Autodesk Inventor part; units mm, degrees
ref_plane "YZ Plane" through (0, 0, 0) normal (1, 0, 0) x (0, 1, 0)
ref_plane "XZ Plane" through (0, 0, 0) normal (0, 1, 0) x (-1, 0, 0)
ref_plane "XY Plane" through (0, 0, 0) normal (0, 0, 1) x (1, 0, 0)
sketch "Skizze1" plane through (0, 0, 0) normal (0, 0, 1) x (1, 0, 0)
  line L0 (-36.5, 103.5) -> (36.5, 103.5)
  line L1 (36.5, 103.5) -> (36.5, -103.5)
  line L2 (36.5, -103.5) -> (-36.5, -103.5)
  line L3 (-36.5, -103.5) -> (-36.5, 103.5)
  point P0 (0, 0)
  point P1 (0, 103.5)
  point P2 (-36.5, 0)
  dimension "d0" = 73
  dimension "d1" = 207
extrude "Extrusion1" add sketch "Skizze1" along normal mid plane 71
sketch "Skizze2" plane through (0, 0, 35.5) normal (0, 0, 1) x (1, 0, 0)
  line L0 (-31.9691, 54.6598) -> (-31.9691, 32.0411)
  line L1 (-31.9691, 32.0411) -> (-18.3639, 32.0411)
  line L2 (-18.3639, 32.0411) -> (-18.3639, 54.6598)
  line L3 (-18.3639, 54.6598) -> (-22.1053, 54.6598)
  line L4 (-22.1053, 54.6598) -> (-22.1053, 35.4424)
  line L5 (-22.1053, 35.4424) -> (-28.2277, 35.4424)
  line L6 (-28.2277, 35.4424) -> (-28.2277, 54.6598)
  line L7 (-28.2277, 54.6598) -> (-31.9691, 54.6598)
  line L8 (-12.2415, 54.6598) -> (-12.2415, 32.0411)
  line L9 (-12.2415, 32.0411) -> (-8.8402, 32.0411)
  line L10 (-8.8402, 32.0411) -> (-8.8402, 40.7145)
  line L11 (-8.8402, 40.7145) -> (-1.8675, 40.7145)
  line L12 (-1.8675, 40.7145) -> (-1.8675, 32.0411)
  line L13 (-1.8675, 32.0411) -> (1.7039, 32.0411)
  line L14 (1.7039, 32.0411) -> (1.7039, 54.6598)
  line L15 (1.7039, 54.6598) -> (-1.8675, 54.6598)
  line L16 (-1.8675, 45.0511) -> (-1.8675, 54.6598)
  line L17 (-1.8675, 45.0511) -> (-8.8402, 45.0511)
  line L18 (-8.8402, 45.0511) -> (-8.8402, 54.6598)
  line L19 (-12.2415, 54.6598) -> (-8.8402, 54.6598)
  line L20 (7.316, 54.6598) -> (7.316, 51.0885)
  line L21 (7.316, 51.0885) -> (12.0779, 51.0885)
  line L22 (12.0779, 51.0885) -> (12.0779, -18.2168)
  line L23 (12.0779, -18.2168) -> (19.2206, -18.2168)
  line L24 (19.2206, -18.2168) -> (19.2206, 51.0885)
  line L25 (19.2206, 51.0885) -> (23.6423, 51.0885)
  line L26 (23.6423, 51.0885) -> (23.6423, 54.6598)
  line L27 (23.6423, 54.6598) -> (7.316, 54.6598)
  line L28 (1.7039, 22.5174) -> (1.7039, 15.0346)
  line L29 (1.7039, 15.0346) -> (29.5946, 15.0346)
  line L30 (29.5946, 15.0346) -> (29.5946, 22.5174)
  line L31 (29.5946, 22.5174) -> (1.7039, 22.5174)
  line L32 (1.7039, -3.1128) -> (29.5946, -3.1128)
  line L33 (29.5946, -3.1128) -> (29.5946, -9.8501)
  line L34 (29.5946, -9.8501) -> (1.7039, -9.8501)
  line L35 (1.7039, -9.8501) -> (1.7039, -3.1128)
  point P0 (0, 0)
  point P1 (12.0779, 22.5174)
  point P2 (12.0779, 15.0346)
  point P3 (19.2206, 15.0346)
  point P4 (19.2206, 22.5174)
  point P5 (19.2206, -3.1128)
  point P6 (19.2206, -9.8501)
  point P7 (12.0779, -9.8501)
  point P8 (12.0779, -3.1128)
extrude "Extrusion2" cut sketch "Skizze2" against normal blind 0.1
chamfer "Fase1" distance 71 angle 15 1 edges at (0, 103.5, 35.5) measured on face at (12.1667, 103.5, -11.8333)
sketch "Skizze3" plane through (-36.5, 84.4756, 35.5) normal (0, 0.9659, 0.2588) x (1, 0, 0)
  circle A0 centre (36.5, 22.9067) radius 15.376
  point P0 (36.5, 12.4265)
extrude "Extrusion3" add sketch "Skizze3" along normal blind 10
properties part number "milch"
Can you work these out from the model? Positions are in its coordinate system, mm. Coordinates: 2 decimals unless noted, no trailing zeros. Loops run counter-clockwise (first coordinate to the right, second up) from the corner with the lowest first, then second, coordinate; pieces in that order, holes last. Notation, with made-up numbers: M 73,37 L 80,37 A15 ccw 80,43 Z; hole C -21,78.25 d10. An arc over 180 degrees is marked long. Return JSON: item names as keys, results as strings. Group by question number.
Item 1: I'm going to push flat-ended pins straight in: pin 1 Ø1.5 at (x, z) = (-27.5, 9.5) entering from +Y; pin 2 Ø6 at (x, z) = (6.5, 17) entering from +Y; pin 3 Ø1 at (x, z) = (-7, -27) entering from +Y. Where does each tip first touch, or does it pass through?
Item 2: Thinking about a two-plate mould opening in Z: for faces 1 (the flat face through (0.51, 95.97, -7.39)), 2 (the flat face through (-1, 1, -35.5)), 3 (the flat face through (36.5, 1, 0)), 4 (the flat face through (-30, 44, 35.4)), which applies, released by +Z, released by -Z, zero draft, split by the parting line, or undercut?
Item 3: If I drill on L1, parallel to Z at x = 15, y = -10.5; L2, parallel to Y at x = -2.5, z = 33.5; L3, parallel to Y at x = -29.5, z = 20.5, over which ranges is the centre line in solid material (lowest first)? Write a range as from..to.
Item 4: Imagine slicing it at B-B (z = -3.5). Please give me the cut outline in (x, y).
Verdict:
{
 "1": {"pin 1": "stops at y = 91.64", "pin 2": "stops at y = 100.59", "pin 3": "stops at y = 101.36"},
 "2": {"face 1": "undercut", "face 2": "released by -Z", "face 3": "zero draft", "face 4": "released by +Z"},
 "3": {"L1": "z = -35.5..35.4", "L2": "y = -103.5..85.01", "L3": "y = -103.5..88.5"},
 "4": {"outline": "M -36.5,-103.5 L 36.5,-103.5 L 36.5,94.93 L -36.5,94.93 Z"}
}
